Design review of the part shown in the three views and the two pictorial views. Dimensions are in mm from the part's minimum x, y and z. A direction names the side the tool comes from. Round coordinates to 2 decimals unless told otherwise and drop trailing zeros. Order: outer loops, then holes, each group sorted by start corner. A loop starts at its lowest first (then second) coordinate and runs counter-clockwise, first axis right, second up.
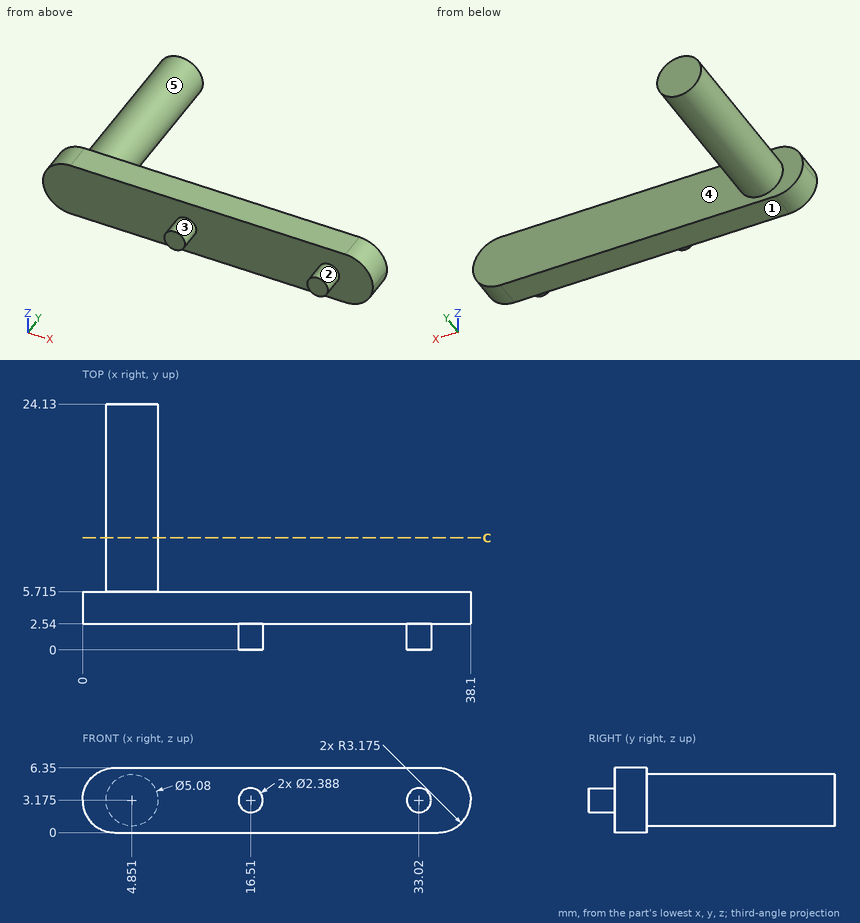
(1) For the marked faces 1 and 2, list the 3-axis set-ups (+Z, -Z, +X, -X, +Y, -Y) from which the entire face can be reached by the end or side of a thin tool; tool diameter is ignored.
Data:
face 1: -Z, +X, -X, +Y, -Y
face 2: -Y
(2) Insertion check: pin 1 (1 mm diameter, centred on y = 15.5, z = 5, fed in from -X) (1 decimal); pin 2 (1 mm diameter, centred on x = 7, z = 5.5, fed in from +Y) (3 decimals); pin 3 (12 mm diameter, centred on x = 17.5, y = 17.5, fed in from -Z); pin 4 (1.5 mm diameter, centred on y = 21.5, z = 2.5, fed in from -X). Each pin has a flat end and moves straight along its axis. Give the tip position at first contact, or say it passes through.
Data:
pin 1: stops at x = 2.7
pin 2: stops at y = 5.715
pin 3: passes through
pin 4: stops at x = 2.31
(3) To check wall thickness, follow probe 1 along Y at (x, z) = (18, 1.75) (1 decimal); probe 2 along Z at (x, y) = (5, 11.75); probe 3 along Y at (x, z) = (6, 3.25). State the ranges of each line that lie inside material, in increasing order.
Data:
probe 1: y = 2.5 to 5.7
probe 2: z = 0.64 to 5.71
probe 3: y = 2.54 to 24.13
(4) Draft analysis for pull direction X (two halves, no side actions). For the marked faces 3, 4 and 5, state which applies: pulls with the +X half, pulls with the -X half, needs draft (parallel to the pull), parting line crosses it, or undercut.
Data:
face 3: undercut
face 4: needs draft
face 5: parting line crosses it
(5) Consider section C-C (y = 11). Write out the cut boundary in (x, z) (1 decimal), and give its area (3 significant figures).
Data:
outline: circle Ø5.1 at (4.9, 3.2)
area: 20.3 mm2
